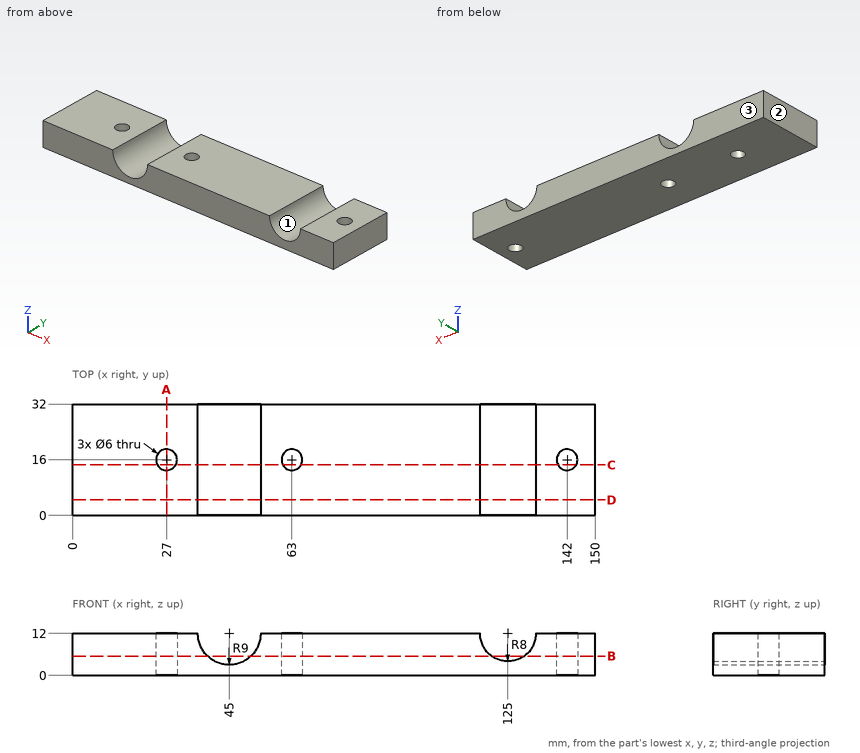
Verification items for this drawing (mm, ordinates from the low corner). Round coordinates to 2 decimals unless told otherwise and drop trailing zeros. Order: outer loops, then holes, each group sorted by start corner. A loop starts at its lowest first (then second) coordinate and runs counter-clockwise, first axis right, second up.
1) Cross-section at C-C, the plane y = 14.5. Record the cut outline in (x, z).
Geometry says:
outline: (0, 0) - (24.4, 0) - (24.4, 12) - (0, 12) - close; (29.6, 0) - (60.4, 0) - (60.4, 12) - (54, 12) arc R9 cw to (36, 12) - (29.6, 12) - close; (65.6, 0) - (139.4, 0) - (139.4, 12) - (133, 12) arc R8 cw to (117, 12) - (65.6, 12) - close; (144.6, 0) - (150, 0) - (150, 12) - (144.6, 12) - close
2) Cross-section at A-A, the plane x = 27. Record the cut outline in (y, z).
Geometry says:
outline: (0, 0) - (13, 0) - (13, 12) - (0, 12) - close; (19, 0) - (32, 0) - (32, 12) - (19, 12) - close
3) Depth check by flat-ended pin: pin 1 (7 mm diameter, centred on x = 63, y = 16, fed in from +Z); pin 2 (5.5 mm diameter, centred on x = 142, y = 16, fed in from +Z). Enter the tip coordinate at first touch or a pass-through.
Geometry says:
pin 1: stops at z = 12
pin 2: passes through
4) Draft check along X on the marked faces 1, 2 and 3. Enter one of: +X half, -X half, draft (parallel to the pull), parting line (faces both ways), or undercut.
Geometry says:
face 1: undercut
face 2: -X half
face 3: draft
5) Cross-section at D-D, the plane y = 4.5. Record the cut outline in (x, z), plus the area to 3 significant figures.
Geometry says:
outline: (0, 0) - (150, 0) - (150, 12) - (133, 12) arc R8 cw to (117, 12) - (54, 12) arc R9 cw to (36, 12) - (0, 12) - close
area: 1,570 mm2
6) Material ranges on line 1 (X direction, y = 7.5, z = 7.75); line 2 (Y direction, x = 63, z = 7); line 3 (X direction, y = 30.5, z = 10.5), recorded low to high.
Geometry says:
line 1: x = 0 to 37.07, 52.93 to 118.22, 131.78 to 150
line 2: y = 0 to 13, 19 to 32
line 3: x = 0 to 36.13, 53.87 to 117.14, 132.86 to 150
7) Cross-section at B-B, the plane z = 5.5. Record the cut outline in (x, y).
Geometry says:
outline: (0, 0) - (38.78, 0) - (38.78, 32) - (0, 32) - close; (51.22, 0) - (120.34, 0) - (120.34, 32) - (51.22, 32) - close; (129.66, 0) - (150, 0) - (150, 32) - (129.66, 32) - close; hole circle Ø6 at (27, 16); hole circle Ø6 at (63, 16); hole circle Ø6 at (142, 16)
